Work out the finished part from the listing and answer in its coordinate system (mm). Round coordinates to 2 decimals unless told otherwise and drop trailing zeros. Write each loop counter-clockwise with the first axis right and the second up, starting at its lowest first coordinate (ties: lowest second). Pieces come first, ordered by that corner, then holes. Notation, with made-up numbers: (-29, 65) - (-6, 65) arc R30 cw to (-6, 101) - close; hole circle Ø3 at (53, 13). An arc over 180 degrees is marked (long way). Answer as a JSON object with one key per item and string values.
```python
from build123d import *

# Parameters (mm, degrees)
SKETCH1_W               = 2
SKETCH1_H               = 6.898115708
BOSS_EXTRUDE1_DEPTH     = 4
SKETCH2_W               = 2
SKETCH2_H               = 4
BOSS_EXTRUDE2_DEPTH     = 23
SKETCH3_W               = 4
SKETCH3_H               = 29.895089618
SKETCH3_R               = 0.5
SKETCH3_W_2             = 1
BOSS_EXTRUDE4_DEPTH     = 2
CUT_EXTRUDE1_DEPTH      = 25.491073296
CUT_EXTRUDE1_DEPTH_BACK = 25.491073296
SKETCH4_R               = 0.5


with BuildPart() as part:
    # Sketch1 → Boss-Extrude1 (new body)
    with BuildSketch(Plane.XY):
        with Locations((0.466430338, -2.557371618)):
            Rectangle(SKETCH1_W, SKETCH1_H)
    extrude(amount=BOSS_EXTRUDE1_DEPTH)

    # Sketch2 → Boss-Extrude2 (add)
    with BuildSketch(Plane(origin=(0, 0.891686236, 0), x_dir=(1, 0, 0), z_dir=(0, 1, 0))):
        with Locations((0.466430338, -2)):
            Rectangle(SKETCH2_W, SKETCH2_H)
    extrude(amount=BOSS_EXTRUDE2_DEPTH)

    # Sketch3 → Boss-Extrude4 (add, through all)
    # profile 1 of 3: a face of its own
    with BuildSketch(Plane(origin=(1.466430338, 0, 0), x_dir=(0, 0, -1), z_dir=(1, 0, 0))):
        with Locations((-2, 8.944141427)):
            Rectangle(SKETCH3_W, SKETCH3_H)
        with Locations((-2, 22.225736667)):
            Circle(SKETCH3_R, mode=Mode.SUBTRACT)
    # profile 2 of 3: a face of its own
    with BuildSketch(Plane(origin=(1.466430338, 0, 0), x_dir=(0, 0, -1), z_dir=(1, 0, 0))):
        with Locations((-4.5, 8.944141427)):
            Rectangle(SKETCH3_W_2, SKETCH3_H)
    # profile 3 of 3: a face of its own
    with BuildSketch(Plane(origin=(1.466430338, 0, 0), x_dir=(0, 0, -1), z_dir=(1, 0, 0))):
        with Locations((0.5, 8.944141427)):
            Rectangle(SKETCH3_W_2, SKETCH3_H)
    extrude(amount=-BOSS_EXTRUDE4_DEPTH)

    # Sketch4 → Cut-Extrude1 (cut, two sides: drawn at the far end of the back side and taken through both)
    with BuildSketch(Plane(origin=(1.466430338, 0, 0), x_dir=(0, 0, -1), z_dir=(1, 0, 0)).offset(-CUT_EXTRUDE1_DEPTH_BACK)):
        with Locations(Location((-2, 22.225736667, 0), (0, 0, 90))):
            Circle(SKETCH4_R)
    extrude(amount=CUT_EXTRUDE1_DEPTH + CUT_EXTRUDE1_DEPTH_BACK, mode=Mode.SUBTRACT)


solid = part.part
```
Item 1: A cutting plane is placed at B-B (y = 22.25). Write down the section's boundary in (x, z), and give its area (3 significant figures).
Results found:
{"outline": "(-0.53, -1) - (1.47, -1) - (1.47, 1.5) - (-0.53, 1.5) - close; (-0.53, 2.5) - (1.47, 2.5) - (1.47, 5) - (-0.53, 5) - close", "area": "10.0 mm²"}
Item 2: This flat-tipped pin is pushed along its axis until it touches: P1, Ø0.5, axis at x = 0, z = 4.5, coming from the -Y side. Where does it stop, or does it pass through?
Results found:
{"P1": "y = -6"}
Item 3: Determine the mould class of faces 1 (the cylindrical face through (0.452, 21.726, 2.022)), 2 (the flat face through (0, 9, -1)), 3 (the flat face through (0, 9, 5)), 4 (the flat face through (-0.534, 9, 2)) for opening direction Z: pulls with the +Z half, pulls with the -Z half, needs draft (parallel to the pull), parting line crosses it, or undercut.
Results found:
{"face 1": "undercut", "face 2": "pulls with the -Z half", "face 3": "pulls with the +Z half", "face 4": "needs draft"}
Item 4: A cutting plane is placed at A-A (z = 2). Write down the section's boundary in (x, y).
Results found:
{"outline": "(-0.53, -6.01) - (1.47, -6.01) - (1.47, 21.73) - (-0.53, 21.73) - close; (-0.53, 22.73) - (1.47, 22.73) - (1.47, 23.89) - (-0.53, 23.89) - close"}
Item 5: Consider line 1 along Y through (x, z) = (0, 2); line 2 along Y through (x, z) = (1, 4.6). Determine where each line is inside the solid, lowest interval first.
Results found:
{"line 1": "-6.01 to 21.73, 22.73 to 23.89", "line 2": "-6 to 23.89"}
